from build123d import *

# Parameters (mm, degrees)
SKETCH1_W                = 1.27
SKETCH1_H                = 2.54
BOSS_EXTRUDE1_DEPTH      = 2.54
SKETCH2_W                = 0.64
SKETCH2_H                = 0.64
BOSS_EXTRUDE2_DEPTH      = 6.1
BOSS_EXTRUDE2_DEPTH_BACK = 5.54


with BuildPart() as part:
    # Sketch1 → Boss-Extrude1 (new body)
    with BuildSketch(Plane(origin=(0, 0, 0), x_dir=(1, 0, 0), z_dir=(0, 1, 0))):
        with Locations((0.635, 1.27)):
            Rectangle(SKETCH1_W, SKETCH1_H)
    extrude(amount=BOSS_EXTRUDE1_DEPTH)

    # Sketch2 → Boss-Extrude2 (add, two sides)
    with BuildSketch(Plane(origin=(0, 2.54, 0), x_dir=(1, 0, 0), z_dir=(0, 1, 0))) as boss_extrude2_sk:
        with Locations((0.635, 1.27)):
            Rectangle(SKETCH2_W, SKETCH2_H)
    extrude(amount=BOSS_EXTRUDE2_DEPTH)
    extrude(boss_extrude2_sk.sketch, amount=-BOSS_EXTRUDE2_DEPTH_BACK)


solid = part.part
Verification items for the finished model (mm, model axes). Coordinates: 2 decimals unless noted, no trailing zeros. Order: outer loops, then holes, each group sorted by start corner. A loop starts at its lowest first (then second) coordinate and runs counter-clockwise, first axis right, second up.
Item 1: Section check C-C, the plane y = 3.5. Enter the section's corners in (x, z) (3 decimals), then the cut area to 3 significant figures.
Filled in:
outline: (0.315, -1.59) - (0.955, -1.59) - (0.955, -0.95) - (0.315, -0.95) - close
area: 0.410 mm2
Item 2: Section check A-A, the plane x = 0.8. Enter the section's corners in (y, z), then the cut area to 3 significant figures.
Filled in:
outline: (-3, -1.59) - (0, -1.59) - (0, -2.54) - (2.54, -2.54) - (2.54, -1.59) - (8.64, -1.59) - (8.64, -0.95) - (2.54, -0.95) - (2.54, 0) - (0, 0) - (0, -0.95) - (-3, -0.95) - close
area: 12.3 mm2
Item 3: Section check B-B, the plane z = -1.1. Enter the section's corners in (x, y) (3 decimals), then the cut area to 3 significant figures.
Filled in:
outline: (0, 0) - (0.315, 0) - (0.315, -3) - (0.955, -3) - (0.955, 0) - (1.27, 0) - (1.27, 2.54) - (0.955, 2.54) - (0.955, 8.64) - (0.315, 8.64) - (0.315, 2.54) - (0, 2.54) - close
area: 9.05 mm2
Item 4: Material ranges on L1, parallel to Y at x = 1.2, z = -2.05; L2, parallel to X at y = 7.75, z = -1 (3 decimals); L3, parallel to Z at x = 0.7, y = 5, recorded low to high.
Filled in:
L1: y = 0 to 2.54
L2: x = 0.315 to 0.955
L3: z = -1.59 to -0.95
Item 5: Depth check by flat-ended pin: pin 1 (0.7 mm diameter, centred on y = 5, z = -1.5, fed in from -X) (3 decimals); pin 2 (0.7 mm diameter, centred on x = 0.5, y = -2, fed in from -Z); pin 3 (0.5 mm diameter, centred on y = -2, z = -1, fed in from +X) (3 decimals). Enter the tip coordinate at first touch or a pass-through.
Filled in:
pin 1: stops at x = 0.315
pin 2: stops at z = -1.59
pin 3: stops at x = 0.955
Item 6: Section check D-D, the plane z = -2.3. Enter the section's corners in (x, y), then the cut area to 3 significant figures.
Filled in:
outline: (0, 0) - (1.27, 0) - (1.27, 2.54) - (0, 2.54) - close
area: 3.23 mm2
